The listing builds one solid part. Answer for the finished solid, in the listing's coordinates (mm). Coordinates: 2 decimals unless noted, no trailing zeros. Order: outer loops, then holes, each group sorted by start corner. A loop starts at its lowest first (then second) coordinate and runs counter-clockwise, first axis right, second up. Notation, with made-up numbers: (-24, 43.5) -> (9, 43.5) arc R8 ccw to (9, 49.5) -> close; hole circle Ø6 at (-25, 5). An arc over 180 degrees is marked (long way). Answer in a Markdown table with one row per item.
Solid Edge part; units mm, degrees
sketch "Sketch1" plane through (0, 0, 0) normal (0, 0, 1) x (1, 0, 0)
  line L0 (-183.0017, -120) -> (-227.4217, -120)
  line L1 (-289.5811, -57.8353) -> (-227.4217, -120)
  line L2 (-289.5811, -57.8353) -> (-351.7458, 4.3295)
  line L3 (-351.7458, 129.7437) -> (-351.7458, 4.3295)
  line L4 (-351.7458, 129.7437) -> (-351.7458, 255.1579)
  line L5 (-289.4346, 317.4691) -> (-351.7458, 255.1579)
  line L6 (-289.4346, 317.4691) -> (-227.7006, 379.2031)
  line L7 (0, 379.2031) -> (-227.7006, 379.2031)
  line L8 (0, 379.2031) -> (0, 0)
  line L9 (0, 0) -> (-183.0017, 0)
  line L10 (-183.0017, 0) -> (-183.0017, -120)
  dimension "D1" = 183.0017
  dimension "D2" = 183.0017
  dimension "D3" = 289.4346
  dimension "D4" = 289.4346
  dimension "D5" = 351.7458
  dimension "D6" = 351.7458
  dimension "D7" = 289.5811
  dimension "D8" = 289.5811
extrude "Protrusion1" add sketch "Sketch1" along normal blind 5
mirror "Mirror1" about plane through (0, 0, 0) normal (1, 0, 0) of "Protrusion1"
sketch "Sketch2" plane through (0, 149.6016, 0) normal (0, 0, -1) x (-1, 0, 0)
  line L0 (-351.7458, -111.1142) -> (-193.1203, -269.6016)
  line L1 (-193.1203, -269.6016) -> (-227.4217, -269.6016)
  arc A0 (-351.7458, -145.2721) -> (-227.4217, -269.6016) centre (-220.2414, -138.0974) ccw
  line L2 (-351.7458, -111.1142) -> (-351.7458, -145.2721)
extrude "Protrusion2" add sketch "Sketch2" against normal up to vertex (5 mm away)
sketch "Sketch3" plane through (0, 149.6016, 0) normal (0, 0, -1) x (-1, 0, 0)
  line L0 (-227.7006, 229.6016) -> (-351.7458, 105.5563)
  arc A0 (-351.7458, 105.5563) -> (-227.7006, 229.6016) centre (-220.2564, 98.1121) cw
extrude "Protrusion3" add sketch "Sketch3" against normal up to vertex (5 mm away)
mirror "Mirror2" about plane through (0, 0, 0) normal (1, 0, 0) of "Protrusion3", "Protrusion2"
sketch "Sketch4" plane through (0, 0, 2.5) normal (0, -1, 0) x (1, 0, 0)
  line L0 (-183.0017, 2.5) -> (183.0017, 2.5)
  line L1 (183.0017, 2.5) -> (183.0017, -2.5)
  line L2 (183.0017, -2.5) -> (-183.0017, -2.5)
  line L3 (-183.0017, -2.5) -> (-183.0017, 2.5)
extrude "Protrusion6" add sketch "Sketch4" along normal blind 1.13
sketch "Sketch5" plane through (0, 129.6016, 5) normal (0, 0, 1) x (1, 0, 0)
  line L0 (-183.0017, -130.7316) -> (183.0017, -130.7316)
  line L1 (183.0017, -130.7316) -> (183.0017, -115.7316)
  line L2 (183.0017, -115.7316) -> (-183.0017, -115.7316)
  line L3 (-183.0017, -115.7316) -> (-183.0017, -130.7316)
  dimension "D1" = 183.0017
extrude "Cutout1" cut sketch "Sketch5" against normal through all
sketch "Sketch6" plane through (0, 129.6016, 5) normal (0, 0, 1) x (1, 0, 0)
  circle A0 centre (-203.0017, -232.7016) radius 3.5
  circle A1 centre (203.0017, -232.7016) radius 3.5
extrude "Cutout2" cut sketch "Sketch6" against normal through all
sketch "Sketch7" plane through (0, 129.6016, 5) normal (0, 0, 1) x (1, 0, 0)
  circle A0 centre (-60, 219.6016) radius 3.5
  circle A1 centre (60, 219.6016) radius 3.5
extrude "Cutout3" cut sketch "Sketch7" against normal through all
properties material "ABS-Plastik, mittelfest"
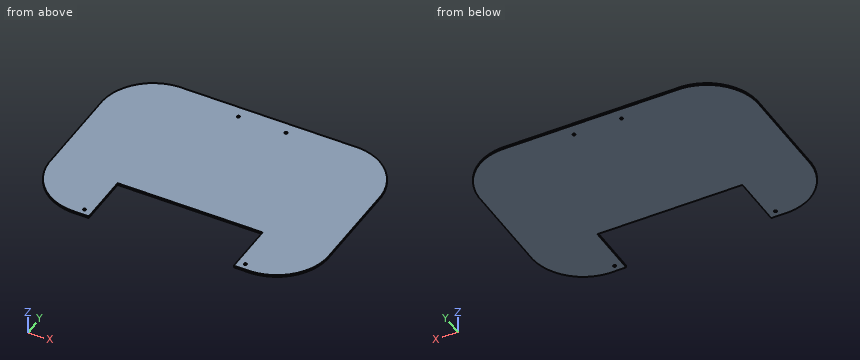
(1) Flat-ended cylindrical pins translate along their axes: pin 1 (3 mm diameter, centred on x = -278, z = 3.5, fed in from +Y); pin 2 (2 mm diameter, centred on x = 234.5, z = 2.5, fed in from +Y); pin 3 (2.5 mm diameter, centred on y = -62.5, z = 3.5, fed in from +X). Find the tip coordinate at first contact, or state that the pin passes through.
Check values:
| item | result |
|---|---|
| pin 1 | y = 366.8 |
| pin 2 | y = 378.75 |
| pin 3 | x = 330.02 |
(2) A cutting plane is placed at A-A, the plane z = 3.55. Determine the outline of the cut face in (x, y), then the cut area to 3 significant figures.
Check values:
| item | result |
|---|---|
| outline | (-351.75, 4.33) arc R131.7 ccw to (-227.42, -120) -> (-183, -120) -> (-183, 13.87) -> (183, 13.87) -> (183, -120) -> (227.42, -120) arc R131.7 ccw to (351.75, 4.33) -> (351.75, 255.16) arc R131.7 ccw to (227.7, 379.2) -> (-227.7, 379.2) arc R131.7 ccw to (-351.75, 255.16) -> close; hole circle Ø7 at (-203, -103.1); hole circle Ø7 at (-60, 349.2); hole circle Ø7 at (60, 349.2); hole circle Ø7 at (203, -103.1) |
| area | 287,000 mm² |
(3) A cutting plane is placed at B-B, the plane x = -298. Determine the outline of the cut face in (y, z).
Check values:
| item | result |
|---|---|
| outline | (-94.79, 0) -> (354.02, 0) -> (354.02, 5) -> (-94.79, 5) -> close |
(4) Find the intervals of material crossed by line 1 along X through (y, z) = (5, 0.55); line 2 along Y through (x, z) = (60, 3.5); line 3 along Y through (x, z) = (-69, 1.8), in increasing order. Write a range as from..to.
Check values:
| item | result |
|---|---|
| line 1 | -351.75..-183, 183..351.75 |
| line 2 | 13.87..345.7, 352.7..379.2 |
| line 3 | 13.87..379.2 |
(5) A cutting plane is placed at C-C, the plane x = 90. Determine the outline of the cut face in (y, z).
Check values:
| item | result |
|---|---|
| outline | (13.87, 0) -> (379.2, 0) -> (379.2, 5) -> (13.87, 5) -> close |
